For this review, take the finished solid that the model builds, in its own axes (mm). Face numbers are marked on the shaded views. Round coordinates to 2 decimals unless told otherwise and drop trailing zeros. Write each loop counter-clockwise with the first axis right and the second up, starting at its lowest first coordinate (ties: lowest second). Pieces come first, ordered by that corner, then holes. Notation, with made-up numbers: M 17.25,-10 L 39.25,-10 A19 cw 39.25,19 Z; hole C -9.5,-2 d11. An arc over 180 degrees is marked long. Answer in a Markdown table with one row per item.
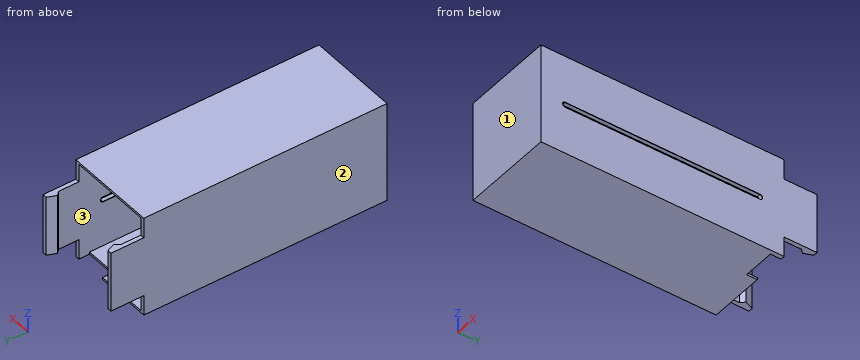
```python
from build123d import *

# Parameters (mm, degrees)
SKETCH1_W           = 38
SKETCH1_H           = 41.8
SKETCH1_W_2         = 34.6
SKETCH1_H_2         = 40
BOSS_EXTRUDE1_DEPTH = 100
SKETCH2_W           = 1.7
SKETCH2_H           = 25
BOSS_EXTRUDE2_DEPTH = 13.6
BOSS_EXTRUDE5_DEPTH = 25
SKETCH6_W           = 38
SKETCH6_H           = 41.8
BOSS_EXTRUDE6_DEPTH = 0.6
SKETCH7_W           = 13.3
SKETCH7_H           = 4.4
CUT_EXTRUDE1_DEPTH  = 10
CUT_EXTRUDE2_DEPTH  = 10
FILLET1_R           = 0.1


with BuildPart() as part:
    # Sketch1 → Boss-Extrude1 (new body)
    with BuildSketch(Plane(origin=(0, 0, 0), x_dir=(1, 0, 0), z_dir=(0, 1, 0))):
        Rectangle(SKETCH1_W, SKETCH1_H)
        Rectangle(SKETCH1_W_2, SKETCH1_H_2, mode=Mode.SUBTRACT)
    extrude(amount=BOSS_EXTRUDE1_DEPTH)

    # Sketch2 → Boss-Extrude2 (add)
    with BuildSketch(Plane(origin=(0, 100, 0), x_dir=(1, 0, 0), z_dir=(0, 1, 0))):
        with Locations((18.15, 0)):
            Rectangle(SKETCH2_W, SKETCH2_H)
        with Locations((-18.15, 0)):
            Rectangle(SKETCH2_W, SKETCH2_H)
    extrude(amount=BOSS_EXTRUDE2_DEPTH)

    # Sketch5 → Boss-Extrude5 (add)
    with BuildSketch(Plane.XY.offset(12.5)):
        Polygon((-15.8, 110), (-17.3, 108.4), (-17.3, 113.6), align=None)
        Polygon((17.3, 108.4), (17.3, 113.6), (15.8, 110), align=None)
    extrude(amount=-BOSS_EXTRUDE5_DEPTH)

    # Sketch6 → Boss-Extrude6 (add)
    with BuildSketch(Plane.XZ):
        Rectangle(SKETCH6_W, SKETCH6_H)
    extrude(amount=BOSS_EXTRUDE6_DEPTH)

    # Sketch7 → Cut-Extrude1 (cut)
    with BuildSketch(Plane(origin=(0, 0, -20.9), x_dir=(-1, 0, 0), z_dir=(0, 0, -1))):
        with Locations((-10.65, 97.8)):
            Rectangle(SKETCH7_W, SKETCH7_H)
    extrude(amount=-CUT_EXTRUDE1_DEPTH, mode=Mode.SUBTRACT)

    # Sketch8 → Cut-Extrude2 (cut)
    with BuildSketch(Plane(origin=(19, 0, 0), x_dir=(0, 0, -1), z_dir=(1, 0, 0))):
        with BuildLine():
            Line((-1, 9.4), (-1, 90))
            ThreePointArc((-1, 90), (0, 91), (1, 90))
            Line((1, 90), (1, 9.4))
            ThreePointArc((1, 9.4), (0, 8.4), (-1, 9.4))
        make_face()
    extrude(amount=-CUT_EXTRUDE2_DEPTH, mode=Mode.SUBTRACT)

    # Fillet1
    fillet1_edges = [part.edges().sort_by_distance(p)[0] for p in [
        (17.3, 49.7, -1),
        (17.3, 91, 0),
        (17.3, 49.7, 1),
        (17.3, 8.4, 0),
        (19, 8.4, 0),
        (19, 49.7, -1),
        (19, 91, 0),
        (19, 49.7, 1),
    ]]
    fillet(fillet1_edges, radius=FILLET1_R)


solid = part.part
```
Q1. Take a section at C-C (z = -3.5). State the section outline as (x, y) points, then the cut area to 3 significant figures.
Found:
| item | result |
|---|---|
| outline | M -19,-0.6 L 19,-0.6 L 19,113.6 L 17.3,113.6 L 15.8,110 L 17.3,108.4 L 17.3,0 L -17.3,0 L -17.3,108.4 L -15.8,110 L -17.3,113.6 L -19,113.6 Z |
| area | 417 mm² |
Q2. For probe 1 along Z at (x, y) = (-1, 15.5); probe 2 along X at (y, z) = (67, -11); probe 3 along Y at (x, z) = (16, -9), list the stretches that pass through material, from the lowest coordinate up.
Found:
| item | result |
|---|---|
| probe 1 | -20.9 to -20, 20 to 20.9 |
| probe 2 | -19 to -17.3, 17.3 to 19 |
| probe 3 | -0.6 to 0, 109.79 to 110.48 |
Q3. Insertion check: P1, Ø1.6, axis at x = -17.5, y = 109, coming from the +Z side; P2, Ø2.5, axis at x = -18, y = 107.5, coming from the -Z side; P3, Ø9, axis at x = 3.5, z = 17, coming from the +Y side. Each pin has a flat end and moves straight along its axis. Give the tip position at first contact, or say it passes through.
Found:
| item | result |
|---|---|
| P1 | z = 12.5 |
| P2 | z = -12.5 |
| P3 | y = 100 |
Q4. Take a section at D-D (x = 7). State the section outline as (y, z) points.
Found:
| item | result |
|---|---|
| outline | M -0.6,-20.9 L 95.6,-20.9 L 95.6,-20 L 0,-20 L 0,20 L 100,20 L 100,20.9 L -0.6,20.9 Z |
Q5. Take a section at A-A (x = -3). State the section outline as (y, z) points.
Found:
| item | result |
|---|---|
| outline | M -0.6,-20.9 L 100,-20.9 L 100,-20 L 0,-20 L 0,20 L 100,20 L 100,20.9 L -0.6,20.9 Z |
Q6. Mouldability with a two-part tool opening along X and no side actions: class the marked faces 1, 2 and 3 as +X half, -X half, draft (parallel to the pull), parting line (faces both ways), or undercut.
Found:
| item | result |
|---|---|
| face 1 | draft |
| face 2 | -X half |
| face 3 | undercut |
Q7. Take a section at B-B (y = 59). State the section outline as (x, z) points, then the cut area to 3 significant figures.
Found:
| item | result |
|---|---|
| outline | M -19,-20.9 L 19,-20.9 L 19,-1.1 A0.1 ccw 18.9,-1 L 17.4,-1 A0.1 ccw 17.3,-1.1 L 17.3,-20 L -17.3,-20 L -17.3,20 L 17.3,20 L 17.3,1.1 A0.1 ccw 17.4,1 L 18.9,1 A0.1 ccw 19,1.1 L 19,20.9 L -19,20.9 Z |
| area | 201 mm² |
